For this review, take the finished solid that the model builds, in its own axes (mm). A direction names the side the tool comes from. Coordinates: 2 decimals unless noted, no trailing zeros. Loops run counter-clockwise (first coordinate to the right, second up) from the corner with the lowest first, then second, coordinate; pieces in that order, holes last. Notation, with made-up numbers: (18.5, 51.25) -> (74.5, 51.25) arc R31 cw to (74.5, 81.25) -> close; hole circle Ø7 at (-11.5, -35). An arc over 180 degrees is marked (long way). Answer in a Markdown table with one row per item.
from build123d import *

# Parameters (mm, degrees)
CABEZA_START            = -2.5
CROQUIS1_R              = 2.25
CABEZA_DEPTH            = 2.5
CROQUIS2_R              = 1.25
CUERPO_DEPTH            = 16
HEXAGONO_INTERIOR_START = -2.5
HEXAGONO_INTERIOR_DEPTH = 1.1


with BuildPart() as part:
    # Croquis1 → Cabeza (new body)
    with BuildSketch(Plane.XY.offset(CABEZA_START)):
        Circle(CROQUIS1_R)
    extrude(amount=CABEZA_DEPTH)

    # Croquis2 → Cuerpo (add)
    with BuildSketch(Plane.XY):
        Circle(CROQUIS2_R)
    extrude(amount=CUERPO_DEPTH)

    # Croquis3 → Hexagono_interior (cut)
    with BuildSketch(Plane.XY.offset(HEXAGONO_INTERIOR_START)):
        Polygon((1.154700538, 0), (0.577350269, 1), (-0.577350269, 1), (-1.154700538, 0), (-0.577350269, -1), (0.577350269, -1), align=None)
    extrude(amount=HEXAGONO_INTERIOR_DEPTH, mode=Mode.SUBTRACT)


solid = part.part
Item 1: Take a section at D-D, the plane y = 1.9. State the section outline as (x, z) points.
Worked answers:
| item | result |
|---|---|
| outline | (-1.21, -2.5) -> (1.21, -2.5) -> (1.21, 0) -> (-1.21, 0) -> close |
Item 2: Take a section at C-C, the plane z = 0.5. State the section outline as (x, y) points.
Worked answers:
| item | result |
|---|---|
| outline | circle Ø2.5 at (0, 0) |
Item 3: For L1, parallel to Z at x = 0.4, y = -0.75; L2, parallel to Z at x = 1.8, y = -0.5; L3, parallel to X at y = 0.1, z = -1, list the stretches that pass through material, from the lowest coordinate up.
Worked answers:
| item | result |
|---|---|
| L1 | -1.4 to 16 |
| L2 | -2.5 to 0 |
| L3 | -2.25 to 2.25 |
Item 4: The part is to be moulded in two halves that separate along Y. For faces 4 (the flat face through (0.86, -0.51, -1.96)), 5 (the cylindrical face through (-0.27, -1.22, 7.89)), 6 (the flat face through (1, 1, -2.5)), say which applies: +Y half, -Y half, draft (parallel to the pull), parting line (faces both ways), or undercut.
Worked answers:
| item | result |
|---|---|
| face 4 | undercut |
| face 5 | parting line |
| face 6 | draft |
Item 5: Take a section at B-B, the plane y = -0.75. State the section outline as (x, z) points, and give its area (3 significant figures).
Worked answers:
| item | result |
|---|---|
| outline | (-2.12, -2.5) -> (-0.72, -2.5) -> (-0.72, -1.4) -> (0.72, -1.4) -> (0.72, -2.5) -> (2.12, -2.5) -> (2.12, 0) -> (1, 0) -> (1, 16) -> (-1, 16) -> (-1, 0) -> (-2.12, 0) -> close |
| area | 41.0 mm² |
Item 6: For faces 1 (the flat face through (1, -1, 0)), 2 (the flat face through (0, 0, 16)), 3 (the flat face through (-0.87, -0.49, -1.96)), list the 3-axis set-ups (+Z, -Z, +X, -X, +Y, -Y) from which the entire face can be reached by the end or side of a thin tool; tool diameter is ignored.
Worked answers:
| item | result |
|---|---|
| face 1 | +Z |
| face 2 | +Z, +X, -X, +Y, -Y |
| face 3 | -Z |
Item 7: Take a section at A-A, the plane x = 0. State the section outline as (y, z) points, and give its area (4 significant figures).
Worked answers:
| item | result |
|---|---|
| outline | (-2.25, -2.5) -> (-1, -2.5) -> (-1, -1.4) -> (1, -1.4) -> (1, -2.5) -> (2.25, -2.5) -> (2.25, 0) -> (1.25, 0) -> (1.25, 16) -> (-1.25, 16) -> (-1.25, 0) -> (-2.25, 0) -> close |
| area | 49.05 mm² |
